Autodesk Inventor part; units mm, degrees
ref_plane "YZ Plane" through (0, 0, 0) normal (1, 0, 0) x (0, 1, 0)
ref_plane "XZ Plane" through (0, 0, 0) normal (0, 1, 0) x (-1, 0, 0)
ref_plane "XY Plane" through (0, 0, 0) normal (0, 0, 1) x (1, 0, 0)
sketch "Sketch2" plane through (0, 0, 0) normal (0, 1, 0) x (-1, 0, 0)
  line L0 (0, 0) -> (44.45, 0)
  line L1 (44.45, 0) -> (44.45, -19.05)
  line L2 (44.45, -19.05) -> (0, -19.05)
  line L3 (0, -19.05) -> (0, 0)
  dimension "d2" = 19.05
  dimension "d3" = 44.45
extrude "Extrusion2" add sketch "Sketch2" along normal blind 25.4
sketch "Sketch6" plane through (0, 25.4, 0) normal (0, 1, 0) x (1, 0, 0)
  line L0 (-44.45, 19.05) -> (-44.45, 0)
  line L1 (-44.45, 9.525) -> (0, 9.525)
  line L2 (0, 0) -> (0, 19.05)
  line L3 (-35.0096, 15.0114) -> (-30.216, 12.3415)
  line L4 (-30.216, 12.3415) -> (-30.1313, 6.8551)
  line L5 (-30.1313, 6.8551) -> (-34.8404, 4.0386)
  line L6 (-34.8404, 4.0386) -> (-39.634, 6.7085)
  line L7 (-39.634, 6.7085) -> (-39.7187, 12.1949)
  line L8 (-39.7187, 12.1949) -> (-35.0096, 15.0114)
  line L9 (-14.3495, 12.1415) -> (-9.6714, 15.0114)
  line L10 (-9.6714, 15.0114) -> (-4.8468, 12.3949)
  line L11 (-4.8468, 12.3949) -> (-4.7005, 6.9085)
  line L12 (-4.7005, 6.9085) -> (-9.3786, 4.0386)
  line L13 (-9.3786, 4.0386) -> (-14.2032, 6.6551)
  line L14 (-14.2032, 6.6551) -> (-14.3495, 12.1415)
  point P0 (-34.925, 9.525)
  point P1 (-9.525, 9.525)
  dimension "d17" = 44.45
  dimension "d18" = 10.9728
  dimension "d19" = 10.9728
  dimension "d20" = 9.525
  dimension "d21" = 9.525
extrude "Extrusion3" cut sketch "Sketch6" against normal blind 8.382
sketch "Sketch17" plane through (0, 0, -19.05) normal (0, 0, -1) x (-1, 0, 0)
  circle A0 centre (22.225, 12.7) radius 3.3782
  line L0 (44.45, 0) -> (44.45, 25.4)
  line L1 (0, 0) -> (44.45, 0)
  dimension "d58" = 22.225
  dimension "d59" = 6.7564
  dimension "d68" = 12.7
extrude "Extrusion11" cut sketch "Sketch17" against normal blind 25.4
sketch "Sketch19" plane through (0, 25.4, 0) normal (0, 1, 0) x (1, 0, 0)
  point P0 (0, 0)
sketch "Sketch20" plane through (0, 25.4, 0) normal (0, 1, 0) x (1, 0, 0)
  line L0 (-4.7005, 6.9085) -> (-9.3786, 4.0386)
  line L1 (-9.3786, 4.0386) -> (-14.2032, 6.6551)
  line L2 (-14.2032, 6.6551) -> (-14.3495, 12.1415)
  line L3 (-14.3495, 12.1415) -> (-9.6714, 15.0114)
  line L4 (-9.6714, 15.0114) -> (-4.8468, 12.3949)
  line L5 (-4.8468, 12.3949) -> (-4.7005, 6.9085)
  line L6 (-14.3495, 12.1415) -> (-9.6714, 15.0114)
  line L7 (-14.2032, 6.6551) -> (-14.3495, 12.1415)
  line L8 (-9.3786, 4.0386) -> (-14.2032, 6.6551)
  line L9 (-4.7005, 6.9085) -> (-9.3786, 4.0386)
  line L10 (-4.8468, 12.3949) -> (-4.7005, 6.9085)
  line L11 (-9.6714, 15.0114) -> (-4.8468, 12.3949)
  line L12 (-30.1313, 6.8551) -> (-34.8404, 4.0386)
  line L13 (-30.216, 12.3415) -> (-30.1313, 6.8551)
  line L14 (-35.0096, 15.0114) -> (-30.216, 12.3415)
  line L15 (-39.7187, 12.1949) -> (-35.0096, 15.0114)
  line L16 (-39.634, 6.7085) -> (-39.7187, 12.1949)
  line L17 (-34.8404, 4.0386) -> (-39.634, 6.7085)
  line L18 (-4.7005, 6.9085) -> (-9.3786, 4.0386)
  line L19 (-9.3786, 4.0386) -> (-9.6714, 15.0114)
  line L20 (-4.8468, 12.3949) -> (-4.7005, 6.9085)
  line L21 (-4.7736, 9.6517) -> (-14.2764, 9.3983)
  line L22 (-14.2032, 6.6551) -> (-14.3495, 12.1415)
  circle A0 centre (-9.525, 9.525) radius 3.3782
  line L23 (-34.8404, 4.0386) -> (-35.0096, 15.0114)
  line L24 (-39.634, 6.7085) -> (-39.7187, 12.1949)
  line L25 (-39.6764, 9.4517) -> (-30.1736, 9.5983)
  line L26 (-30.216, 12.3415) -> (-30.1313, 6.8551)
  circle A1 centre (-34.925, 9.525) radius 3.3782
  point P0 (0, 0)
  dimension "d64" = 6.7564
  dimension "d65" = 6.7564
extrude "Extrusion12" cut sketch "Sketch20" against normal through all contours A0 L21 L19 | L19 L21 A0 | L21 L19 A0 | L21 A0 L19 | A1 L25 L23 | L23 L25 A1 | L25 L23 A1 | L25 A1 L23
sketch "Sketch21" plane through (0, 25.4, 0) normal (0, 1, 0) x (1, 0, 0)
  point P0 (0, 0)
properties part number "bumper piece 1"
Work out the finished part from the listing and answer in its coordinate system (mm). A direction names the side the tool comes from. Give positions to 0.01 mm unless a question says otherwise; leave off trailing zeros. Order: outer loops, then holes, each group sorted by start corner. A loop starts at its lowest first (then second) coordinate and runs counter-clockwise, first axis right, second up. Notation, with made-up numbers: M 36,-34 L 83,-34 A21 cw 83,-24 Z; hole C -10,43.25 d6. An arc over 180 degrees is marked long. Return JSON: item names as keys, results as strings.
Q1. The mould has two halves that part along Z. Classify faces 3 (the face through (-7.29, 21.27, -13.72)), 4 (the face through (-27, 13, 0)), 5 (the face through (-18, 13, -19.05)): pulls with the +Z half, pulls with the -Z half, needs draft (parallel to the pull), parting line crosses it, or undercut.
Answer below:
{"face 3": "undercut", "face 4": "pulls with the +Z half", "face 5": "pulls with the -Z half"}
Q2. Find section A-A, the plane y = 14.25. Write down the section's boundary in (x, z) (3 decimals).
Answer below:
{"outline": "M -44.45,-19.05 L -25.227,-19.05 L -25.227,0 L -44.45,0 Z; M -19.223,-19.05 L 0,-19.05 L 0,0 L -19.223,0 Z; hole C -34.925,-9.525 d6.756; hole C -9.525,-9.525 d6.756"}
Q3. Find the intervals of material crossed by line 1 along Y through (x, z) = (-22.5, -3.75); line 2 along X through (y, z) = (3.5, -7.5); line 3 along X through (y, z) = (10.25, -12), in increasing order. Write a range as [from, to].
Answer below:
{"line 1": "y = [0, 9.33], [16.07, 25.4]", "line 2": "x = [-44.45, -37.63], [-32.22, -12.23], [-6.82, 0]", "line 3": "x = [-44.45, -37.22], [-32.63, -24.55], [-19.9, -11.82], [-7.23, 0]"}
Q4. This flat-tipped pin is pushed along its axis until it touches: pin 1 (10.5 mm diameter, centred on x = -35, z = -11.5, fed in from +Y). Where does it stop, or does it pass through?
Answer below:
{"pin 1": "stops at y = 25.4"}
Q5. Find section C-C, the plane x = -21. Write down the section's boundary in (y, z).
Answer below:
{"outline": "M 0,-19.05 L 9.55,-19.05 L 9.55,0 L 0,0 Z; M 15.85,-19.05 L 25.4,-19.05 L 25.4,0 L 15.85,0 Z"}
Q6. Find section D-D, the plane y = 10. Write down the section's boundary in (x, z) (3 decimals), and give its area (3 significant figures).
Answer below:
{"outline": "M -44.45,-19.05 L -24.255,-19.05 L -24.255,0 L -44.45,0 Z; M -20.195,-19.05 L 0,-19.05 L 0,0 L -20.195,0 Z; hole C -34.925,-9.525 d6.756; hole C -9.525,-9.525 d6.756", "area": "698 mm^2"}
Q7. Which of the six approach directions +Z, -Z, +X, -X, +Y, -Y give full straight-line access (tool end or side, diameter ignored) to faces 1 (the face through (-19.544, 10.644, -9.658)), 2 (the face through (-37.4, 21.27, -13.58))?
Answer below:
{"face 1": "+Z, -Z", "face 2": "+Y"}
Q8. Find section B-B, the plane z = -3. Write down the section's boundary in (x, y) (3 decimals), and give its area (3 significant figures).
Answer below:
{"outline": "M -44.45,0 L 0,0 L 0,25.4 L -44.45,25.4 Z; hole C -22.225,12.7 d6.756", "area": "1,090 mm^2"}
